The listing builds one solid part. Answer for the finished solid, in the listing's coordinates (mm). Face numbers are marked on the shaded views. A direction names the side the tool comes from. Round coordinates to 2 decimals unless told otherwise and drop trailing zeros. Order: outer loops, then holes, each group sorted by start corner. A loop starts at its lowest first (then second) coordinate and runs counter-clockwise, first axis right, second up. Notation, with made-up numbers: (72, -8.5) -> (104, -8.5) arc R18 cw to (104, 8.5) -> close; hole circle Ø10 at (-36.5, -25.75). An arc over 180 degrees is marked (long way). Return JSON: item names as keys, results as strings. Group by question number.
(1) The part is cut by section B-B (z = 0). Determine the outline of the cut face in (x, y), plus the area to 3 significant figures.
(2) The part is cut by section D-D (y = -7.5). Determine the outline of the cut face in (x, z).
(3) Determine the mould class of the marked faces 5, 6 and 7 for opening direction Z: +Z half, -Z half, draft (parallel to the pull), parting line (faces both ways), or undercut.
(4) The part is cut by section C-C (x = 105.5). Determine the outline of the cut face in (y, z), plus the area to 3 significant figures.
(5) Consider line 1 (X direction, y = -23, z = 8.5); line 2 (Z direction, x = 15, y = -10); line 3 (Z direction, x = 15, y = 23). Determine where each line is inside the solid, lowest interval first. Write a range as [from, to].
(6) Which of the six approach directions +Z, -Z, +X, -X, +Y, -Y give full straight-line access (tool end or side, diameter ignored) to the marked faces 1, 2, 3 and 4?
(7) The part is cut by section A-A (y = -19). Determine the outline of the cut face in (x, z).
(8) Each of these flat-tipped pins is pushed along its axis until it touches: pin 1 (5 mm diameter, centred on x = 60.5, z = 56, fed in from +Y); pin 2 (4.5 mm diameter, centred on x = 133.5, y = 26, fed in from +Z); pin 3 (3 mm diameter, centred on x = 37.5, y = -21.5, fed in from +Z). Where does it stop, or does it pass through?
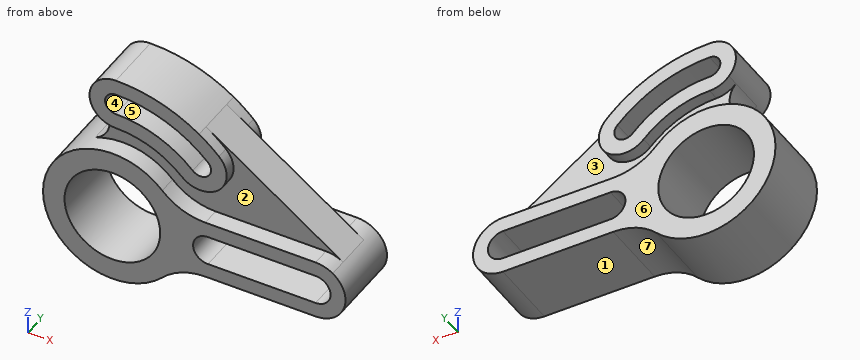
from build123d import *

# Parameters (mm, degrees)
F1_DEPTH = 15
F0_R     = 40
F2_DEPTH = 30
F3_DEPTH = 25
F4_DEPTH = 25


with BuildPart() as f1:
    # F0 (on Front) → F1 (new body, symmetric)
    with BuildSketch(Plane.XZ):
        with BuildLine():
            ThreePointArc((55.1543289326, 55.1543289326), (29.8493077245, 72.0626035359), (0, 78))
            ThreePointArc((0, 78), (-8.8522259778, 79.8595408384), (-16.2079905268, 85.1238095238))
            ThreePointArc((-16.2079905268, 85.1238095238), (-11.3825323132, 67.4278790278), (-23.0085459926, 53.241025641))
            ThreePointArc((-23.0085459926, 53.241025641), (11.3872373178, 56.8711774651), (41.7336868403, 40.2777777778))
            ThreePointArc((41.7336868403, 40.2777777778), (58.1676040827, 28.9776624284), (77.7110030819, 25))
            Line((77.7110030819, 25), (170, 25))
            ThreePointArc((170, 25), (177.4741993043, 23.8565786474), (184.2647058824, 20.5309075808))
            Line((184.2647058824, 20.5309075808), (69.6117647059, 100.1908289941))
            ThreePointArc((69.6117647059, 100.1908289941), (78.2497125429, 93.6001201225), (86.2670273048, 86.2670273048))
            ThreePointArc((86.2670273048, 86.2670273048), (86.2670273048, 55.1543289326), (55.1543289326, 55.1543289326))
        make_face()
    extrude(amount=F1_DEPTH, both=True)

    # F0 (on Front) → F2 (join, symmetric)
    with BuildSketch(Plane.XZ):
        with BuildLine():
            ThreePointArc((41.7336868403, 40.2777777778), (11.3872373178, 56.8711774651), (-23.0085459926, 53.241025641))
            ThreePointArc((-23.0085459926, 53.241025641), (-47.6875180017, -33.013643041), (41.7336868403, -40.2777777778))
            ThreePointArc((41.7336868403, -40.2777777778), (58.1676040827, -28.9776624284), (77.7110030819, -25))
            Line((77.7110030819, -25), (170, -25))
            ThreePointArc((170, -25), (193.8565786474, -7.4741993043), (184.2647058824, 20.5309075808))
            ThreePointArc((184.2647058824, 20.5309075808), (177.4741993043, 23.8565786474), (170, 25))
            Line((170, 25), (77.7110030819, 25))
            ThreePointArc((77.7110030819, 25), (58.1676040827, 28.9776624284), (41.7336868403, 40.2777777778))
        make_face()
        Circle(F0_R, mode=Mode.SUBTRACT)
        with BuildLine():
            Line((170, -12.5), (80, -12.5))
            ThreePointArc((80, -12.5), (67.5, 0), (80, 12.5))
            Line((80, 12.5), (170, 12.5))
            ThreePointArc((170, 12.5), (182.5, 0), (170, -12.5))
        make_face(mode=Mode.SUBTRACT)
    extrude(amount=F2_DEPTH, both=True)

    # F0 (on Front) → F3 (join, symmetric)
    with BuildSketch(Plane.XZ):
        with BuildLine():
            ThreePointArc((-16.2079905268, 85.1238095238), (-8.8522259778, 79.8595408384), (0, 78))
            ThreePointArc((0, 78), (29.8493077245, 72.0626035359), (55.1543289326, 55.1543289326))
            ThreePointArc((55.1543289326, 55.1543289326), (86.2670273048, 55.1543289326), (86.2670273048, 86.2670273048))
            ThreePointArc((86.2670273048, 86.2670273048), (78.2497125429, 93.6001201225), (69.6117647059, 100.1908289941))
            ThreePointArc((69.6117647059, 100.1908289941), (36.474092605, 116.4201037993), (0, 122))
            ThreePointArc((0, 122), (-20.1404591616, 108.8522259778), (-16.2079905268, 85.1238095238))
        make_face()
        with BuildLine():
            ThreePointArc((64.346717088, 64.346717088), (34.8241923452, 84.0730374585), (0, 91))
            ThreePointArc((0, 91), (-9, 100), (0, 109))
            ThreePointArc((0, 109), (41.7124941278, 100.7028690437), (77.0746391493, 77.0746391493))
            ThreePointArc((77.0746391493, 77.0746391493), (77.0746391493, 64.346717088), (64.346717088, 64.346717088))
        make_face(mode=Mode.SUBTRACT)
    extrude(amount=F3_DEPTH, both=True)

    # F0 (on Front) → F4 (join, symmetric)
    with BuildSketch(Plane.XZ):
        with BuildLine():
            ThreePointArc((-16.2079905268, 85.1238095238), (-8.8522259778, 79.8595408384), (0, 78))
            ThreePointArc((0, 78), (29.8493077245, 72.0626035359), (55.1543289326, 55.1543289326))
            ThreePointArc((55.1543289326, 55.1543289326), (86.2670273048, 55.1543289326), (86.2670273048, 86.2670273048))
            ThreePointArc((86.2670273048, 86.2670273048), (78.2497125429, 93.6001201225), (69.6117647059, 100.1908289941))
            ThreePointArc((69.6117647059, 100.1908289941), (36.474092605, 116.4201037993), (0, 122))
            ThreePointArc((0, 122), (-20.1404591616, 108.8522259778), (-16.2079905268, 85.1238095238))
        make_face()
        with BuildLine():
            ThreePointArc((64.346717088, 64.346717088), (34.8241923452, 84.0730374585), (0, 91))
            ThreePointArc((0, 91), (-9, 100), (0, 109))
            ThreePointArc((0, 109), (41.7124941278, 100.7028690437), (77.0746391493, 77.0746391493))
            ThreePointArc((77.0746391493, 77.0746391493), (77.0746391493, 64.346717088), (64.346717088, 64.346717088))
        make_face(mode=Mode.SUBTRACT)
    extrude(amount=F4_DEPTH, both=True)


solid = f1.part
Answer below:
{
 "1": {"outline": "(-58, -30) -> (-40, -30) -> (-40, 30) -> (-58, 30) -> close; (40, -30) -> (67.5, -30) -> (67.5, 30) -> (40, 30) -> close; (182.5, -30) -> (195, -30) -> (195, 30) -> (182.5, 30) -> close", "area": "3,480 mm²"},
 "2": {"outline": "(-23.01, 53.24) arc R58 ccw (long way) to (41.73, -40.28) arc R50 cw to (77.71, -25) -> (170, -25) arc R25 ccw to (184.26, 20.53) -> (69.61, 100.19) arc R122 ccw to (0, 122) arc R22 ccw to (-16.21, 85.12) arc R20 cw to start; hole circle Ø80 at (0, 0); hole (0, 91) arc R91 cw to (64.35, 64.35) arc R9 ccw to (77.07, 77.07) arc R109 ccw to (0, 109) arc R9 ccw to start; hole (80, -12.5) -> (170, -12.5) arc R12.5 ccw to (170, 12.5) -> (80, 12.5) arc R12.5 ccw to start"},
 "3": {"face 5": "undercut", "face 6": "draft", "face 7": "-Z half"},
 "4": {"outline": "(-30, -25) -> (30, -25) -> (30, -12.5) -> (-30, -12.5) -> close; (-30, 12.5) -> (30, 12.5) -> (30, 25) -> (15, 25) -> (15, 75.26) -> (-15, 75.26) -> (-15, 25) -> (-30, 25) -> close", "area": "3,010 mm²"},
 "5": {"line 1": "x = [-57.37, -39.09], [39.09, 70.83], [179.17, 193.51]", "line 2": "z = [-56.03, -37.08], [37.08, 89.76], [107.96, 121.07]", "line 3": "z = [-56.03, -37.08], [37.08, 56.03], [76.54, 89.76], [107.96, 121.07]"},
 "6": {"face 1": "-Z, +X, +Y, -Y", "face 2": "-Y", "face 3": "+Y", "face 4": "+Y, -Y"},
 "7": {"outline": "(0, 78) arc R78 cw to (55.15, 55.15) arc R22 ccw to (86.27, 86.27) arc R122 ccw to (0, 122) arc R22 ccw to start; (41.73, -40.28) arc R50 cw to (77.71, -25) -> (170, -25) arc R25 ccw to (170, 25) -> (77.71, 25) arc R50 cw to (41.73, 40.28) arc R58 ccw (long way) to start; hole circle Ø80 at (0, 0); hole (0, 91) arc R91 cw to (64.35, 64.35) arc R9 ccw to (77.07, 77.07) arc R109 ccw to (0, 109) arc R9 ccw to start; hole (80, -12.5) -> (170, -12.5) arc R12.5 ccw to (170, 12.5) -> (80, 12.5) arc R12.5 ccw to start"},
 "8": {"pin 1": "stops at y = 25", "pin 2": "stops at z = 25", "pin 3": "stops at z = 116.57"}
}
